Answer from the drawing. Dimensions are ordinates in mm from the lowest x, y and z of the part. Coordinates: 2 decimals unless noted, no trailing zeros. Loops run counter-clockwise (first coordinate to the right, second up) from the corner with the lowest first, then second, coordinate; pieces in that order, holes last. Notation, with made-up numbers: (24, 40) - (64, 40) arc R18 cw to (64, 49) - close; hole circle Ø7 at (20.5, -13). An arc over 180 degrees is marked (long way). One line per question, with ' | ' between items. Start each with the question number.
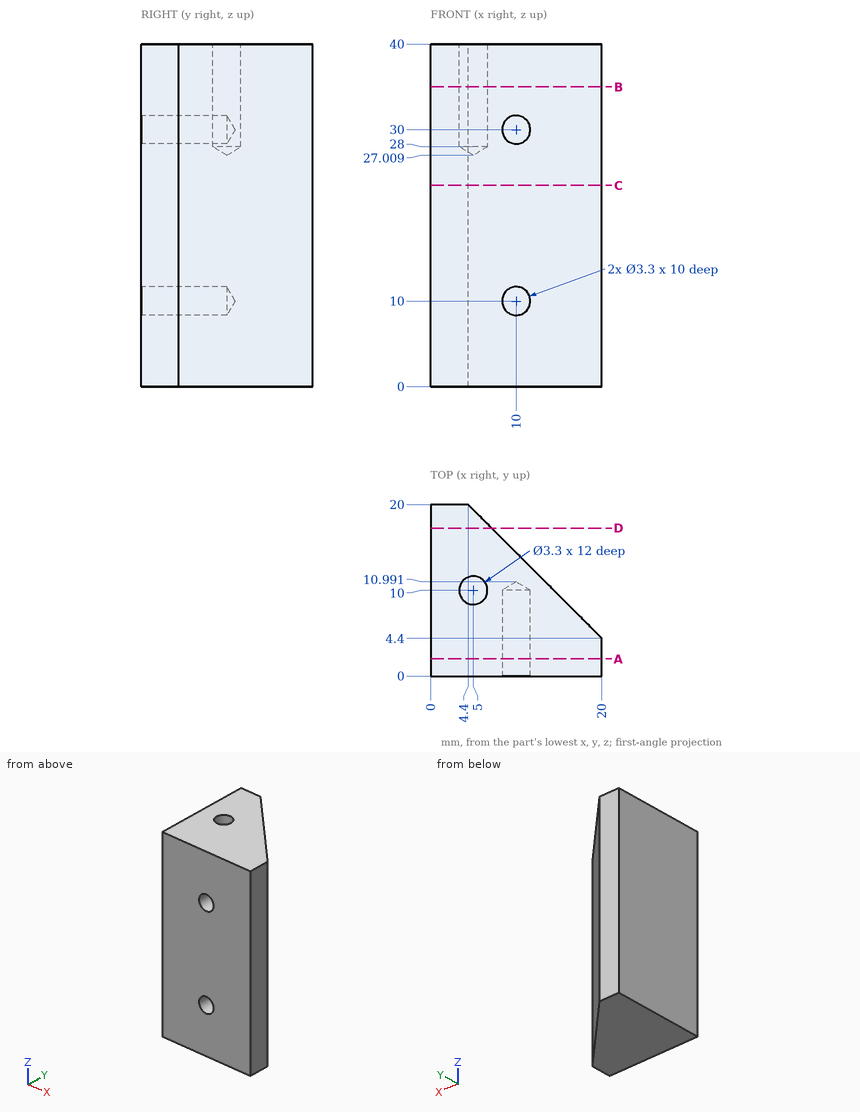
1) The part is cut by section A-A on y = 2. Write down the section's boundary in (x, z).
2) Find the intervals of material crossed by line 1 along Z through (x, y) = (10, 6.75); line 2 along Y through (x, z) = (5, 33); line 3 along X through (y, z) = (12.75, 4), in increasing order. Write a range as from..to.
3) The part is cut by section C-C on z = 23.5. Write down the section's boundary in (x, y), and give its area (3 significant figures).
4) The part is cut by section D-D on y = 17.25. Write down the section's boundary in (x, z).
5) Given pin 1 Ø8 at (y, z) = (10, 26.5) entering from +X; pin 2 Ø2.5 at (x, y) = (5, 10) entering from +Z; pin 3 Ø4 at (x, z) = (10, 10) entering from +Y, each flat-ended and moving along its own axis, determine where each tip first touches the part or whether it passes through.
6) The part is cut by section B-B on z = 35. Write down the section's boundary in (x, y), and give its area (3 significant figures).
Answer below:
1) outline: (0, 0) - (20, 0) - (20, 40) - (0, 40) - close; hole circle Ø3.3 at (10, 10); hole circle Ø3.3 at (10, 30)
2) line 1: 0..8.35, 11.65..28.35, 31.65..40 | line 2: 0..8.35, 11.65..19.4 | line 3: 0..11.65
3) outline: (0, 0) - (20, 0) - (20, 4.4) - (4.4, 20) - (0, 20) - close | area: 278 mm2
4) outline: (0, 0) - (7.15, 0) - (7.15, 40) - (0, 40) - close
5) pin 1: x = 18.4 | pin 2: z = 27.76 | pin 3: y = 16.4
6) outline: (0, 0) - (20, 0) - (20, 4.4) - (4.4, 20) - (0, 20) - close; hole circle Ø3.3 at (5, 10) | area: 270 mm2
